Could you check a few things on this model? Use its own coordinates, in mm. A direction names the side the tool comes from. Give positions to 0.01 mm unless a question says otherwise; leave off trailing zeros. Order: outer loops, then holes, each group sorted by start corner. A loop starts at its lowest first (then second) coordinate and runs counter-clockwise, first axis right, second up. Notation, with made-up numbers: (86.25, 21.5) - (130.25, 21.5) arc R23 ccw to (130.25, 54.5) - close; hole circle Ø8 at (64, 51.5). An arc over 180 degrees is marked (long way). Put each result on its own line as item: value.
from build123d import *

# Parameters (mm, degrees)
SKETCH1_R                          = 31.5
BOSS_EXTRUDE1_DEPTH                = 21
TAP_DRILL_FOR_M2_5X0_45_TAP2_D     = 2.05
TAP_DRILL_FOR_M2_5X0_45_TAP2_DEPTH = 7
TAP_DRILL_FOR_M2_5X0_45_TAP2_TIP   = 0.615882135
SKETCH6_R                          = 27
CUT_EXTRUDE1_DEPTH                 = 10


with BuildPart() as part:
    # Sketch1 → Boss-Extrude1 (new body)
    with BuildSketch(Plane(origin=(0, 0, 0), x_dir=(1, 0, 0), z_dir=(0, 1, 0))):
        Circle(SKETCH1_R)
    extrude(amount=BOSS_EXTRUDE1_DEPTH)

    # Tap Drill for M2.5x0.45 Tap2
    with Locations(Plane(origin=(0, 21, 0), x_dir=(1, 0, 0), z_dir=(0, 1, 0))):
        with Locations((-5.303300859, 5.303300859), (5.303300859, 5.303300859), (5.303300859, -5.303300859), (-5.303300859, -5.303300859)):
            Hole(TAP_DRILL_FOR_M2_5X0_45_TAP2_D / 2, depth=TAP_DRILL_FOR_M2_5X0_45_TAP2_DEPTH)
            with Locations((0, 0, -(TAP_DRILL_FOR_M2_5X0_45_TAP2_DEPTH + TAP_DRILL_FOR_M2_5X0_45_TAP2_TIP / 2))):  # 118° drill point
                Cone(0, TAP_DRILL_FOR_M2_5X0_45_TAP2_D / 2, TAP_DRILL_FOR_M2_5X0_45_TAP2_TIP, mode=Mode.SUBTRACT)

    # Sketch6 → Cut-Extrude1 (cut)
    with BuildSketch(Plane.XZ):
        Circle(SKETCH6_R)
    extrude(amount=-CUT_EXTRUDE1_DEPTH, mode=Mode.SUBTRACT)


solid = part.part
1) I'm going to push flat-ended pins straight in: pin 1 (1.6 mm diameter, centred on x = -5.3, z = -5.3, fed in from -Y); pin 2 (4 mm diameter, centred on y = 3.5, z = -25, fed in from +X); pin 3 (2 mm diameter, centred on x = -13, y = 12.5, fed in from -Z). Where does each tip first touch, or does it pass through?
Filled in:
pin 1: stops at y = 10
pin 2: stops at x = 21.52
pin 3: stops at z = -29.12
2) Which directions (+Z, -Z, +X, -X, +Y, -Y) give clear straight access to the entire face, cutting with the end or side of a thin tool? Please do faces 1 (the cylindrical face through (-5.85, 4.93, -26.36)), 2 (the flat face through (0, 21, 0)), 3 (the cylindrical face through (-4.55, 17.45, 4.61)).
Filled in:
face 1: -Y
face 2: +Z, -Z, +X, -X, +Y
face 3: +Y
3) Suppose I cut it at A-A, the plane x = 0. List the corners of the cut face in (y, z) for me.
Filled in:
outline: (0, -31.5) - (21, -31.5) - (21, 31.5) - (0, 31.5) - (0, 27) - (10, 27) - (10, -27) - (0, -27) - close
4) Suppose I cut it at D-D, the plane y = 5.5. List the corners of the cut face in (x, z) for me, and give its area (3 significant figures).
Filled in:
outline: circle Ø63 at (0, 0); hole circle Ø54 at (0, 0)
area: 827 mm^2
5) We'd pull the mould along Z, two halves only. Please class faces 4 (the cylindrical face through (-4.101, 10.353, -31.232)), 5 (the flat face through (0, 10, 0)), 6 (the flat face through (23.19, 0, -14.15)): pulls with the +Z half, pulls with the -Z half, needs draft (parallel to the pull), parting line crosses it, or undercut.
Filled in:
face 4: parting line crosses it
face 5: undercut
face 6: needs draft
6) Suppose I cut it at B-B, the plane z = 0. List the corners of the cut face in (x, y) for me.
Filled in:
outline: (-31.5, 0) - (-27, 0) - (-27, 10) - (27, 10) - (27, 0) - (31.5, 0) - (31.5, 21) - (-31.5, 21) - close
7) Suppose I cut it at C-C, the plane y = 18.5. List the corners of the cut face in (x, z) for me (3 decimals).
Filled in:
outline: circle Ø63 at (0, 0); hole circle Ø2.05 at (-5.303, -5.303); hole circle Ø2.05 at (-5.303, 5.303); hole circle Ø2.05 at (5.303, -5.303); hole circle Ø2.05 at (5.303, 5.303)
8) If I drill on line 1 (X direction, y = 14.25, z = 5); line 2 (Y direction, x = -2, z = -7); line 3 (Z direction, x = 0.5, y = 14.5), over which ranges is the centre line in solid material (lowest first)? Write a range as [from, to].
Filled in:
line 1: x = [-31.1, -6.28], [-4.32, 4.32], [6.28, 31.1]
line 2: y = [10, 21]
line 3: z = [-31.5, 31.5]
